Read the model definition and answer for the solid it produces. Units are mm, in the model's axes. A direction names the side the tool comes from. Round coordinates to 2 decimals unless told otherwise and drop trailing zeros. Write each loop counter-clockwise with the first axis right and the second up, starting at its lowest first coordinate (ties: lowest second). Pieces come first, ordered by that corner, then holes. Notation, with made-up numbers: (53, 60) - (92, 60) arc R21 cw to (92, 97) - close; hole circle Ø2 at (-21, 61). An arc over 180 degrees is marked (long way). One line per item, written item: value. Start each with the question number.
(1) A cutting plane is placed at A-A, the plane z = 6.75. Determine the outline of the cut face in (x, y).
(2) Find the intervals of material crossed by L1, parallel to Z at x = -2.5, y = 4; L2, parallel to Y at x = 9, z = 12.5; L3, parallel to Y at x = 12, z = 17.5, in increasing order.
(3) For faces 1 (the face through (5.989, -11.544, 22.712)), 2 (the face through (5.989, 11.544, 22.712)), 3 (the face through (-2.25, 0, 7)), determine the directions among +Z, -Z, +X, -X, +Y, -Y from which every point of the face is accessible in a straight line to the end or side of a thin tool.
(4) A cutting plane is placed at B-B, the plane x = 13. Determine the outline of the cut face in (y, z).
(5) A cutting plane is placed at C-C, the plane z = 11. Determine the outline of the cut face in (x, y).
(6) Flat-ended cylindrical pins translate along their axes: pin 1 Ø1.6 at (y, z) = (-6.5, 23) entering from +X; pin 2 Ø3 at (y, z) = (-4, 7.5) entering from -X; pin 3 Ø6 at (y, z) = (4, 6) entering from +X. Find the tip coordinate at first contact, or state that the pin passes through.
(7) The mould has two halves that part along Z. Classify faces 4 (the face through (12.671, -11.854, 14.79)), 5 (the face through (-5.989, 11.544, 22.712)), 6 (the face through (0, 0, 0)): +Z half, -Z half, draft (parallel to the pull), parting line (faces both ways), or undercut.
(8) A cutting plane is placed at D-D, the plane y = 9.5. Determine the outline of the cut face in (x, z).
from build123d import *

# Parameters (mm, degrees)
F1_DEPTH     = 30
F2_W         = 2.5
F2_H         = 5.5
F3_DEPTH     = 27
F4_T1_DEPTH  = 68.7298334621
F5_T1_DEPTH  = 5.5
F5_T3_DEPTH  = 5.5
F5_T8_DEPTH  = 30.5
F5_T13_DEPTH = 30.5
F5_T18_DEPTH = 30.5
F5_T23_DEPTH = 30.5
F5_T28_DEPTH = 30.5
F5_T33_DEPTH = 30.5
F5_T38_DEPTH = 30.5
F5_T43_DEPTH = 30.5


# Not quite as in the source:
# - a fillet or chamfer that OpenCascade refuses, or shapes differently, is made with other operations: its cross-section is extruded or revolved along the edge and cut away or added


with BuildPart() as f1:
    # F0 (on Top) → F1 (new body)
    with BuildSketch(Plane.XY):
        with BuildLine():
            Line((15.75, 13.25), (-15.75, 13.25))
            Line((-15.75, 13.25), (-15.75, 8.25))
            ThreePointArc((-15.75, 8.25), (-9.9163690552, 5.8336309448), (-7.5, 0))
            ThreePointArc((-7.5, 0), (-9.9163690552, -5.8336309448), (-15.75, -8.25))
            Line((-15.75, -8.25), (-15.75, -13.25))
            Line((-15.75, -13.25), (15.75, -13.25))
            Line((15.75, -13.25), (15.75, -8.25))
            ThreePointArc((15.75, -8.25), (7.5, 0), (15.75, 8.25))
            Line((15.75, 8.25), (15.75, 13.25))
        make_face()
    extrude(amount=F1_DEPTH)

    # F2 (on face) → F3 (cut)
    with BuildSketch(Plane.XZ.offset(13.25)):
        with Locations((-3.5, 22.75)):
            Rectangle(F2_W, F2_H)
        with Locations((-3.5, 7.25)):
            Rectangle(F2_W, F2_H)
        with Locations((3.5, 22.75)):
            Rectangle(F2_W, F2_H)
        with Locations((3.5, 7.25)):
            Rectangle(F2_W, F2_H)
    extrude(amount=-F3_DEPTH, mode=Mode.SUBTRACT)

    # F4: fillet of radius 8.5 on 4 edges, made by hand

    # F4_s2 → F4_t1 (cut)
    with BuildSketch(Plane.XY.offset(-19.364916731)):
        with BuildLine():
            ThreePointArc((-8.0040333076, 13.25), (-12.6138055362, 11.8914284285), (-15.75, 8.25))
            Line((-15.75, 8.25), (-15.75, 13.25))
            Line((-15.75, 13.25), (-8.0040333076, 13.25))
        make_face()
        with BuildLine():
            ThreePointArc((-8.0040333076, -13.25), (-12.6138055362, -11.8914284285), (-15.75, -8.25))
            Line((-15.75, -8.25), (-15.75, -13.25))
            Line((-15.75, -13.25), (-8.0040333076, -13.25))
        make_face()
        with BuildLine():
            ThreePointArc((15.75, -8.25), (12.6138055362, -11.8914284285), (8.0040333076, -13.25))
            Line((8.0040333076, -13.25), (15.75, -13.25))
            Line((15.75, -13.25), (15.75, -8.25))
        make_face()
        with BuildLine():
            ThreePointArc((15.75, 8.25), (12.6138055362, 11.8914284285), (8.0040333076, 13.25))
            Line((8.0040333076, 13.25), (15.75, 13.25))
            Line((15.75, 13.25), (15.75, 8.25))
        make_face()
    extrude(amount=F4_T1_DEPTH, mode=Mode.SUBTRACT)

    # F5: fillet of radius 5 on 8 edges, made by hand

    # F5_s2 → F5_t1 (cut)
    with BuildSketch(Plane.XY.offset(20)):
        with BuildLine():
            ThreePointArc((-9.75, -13.25), (-6.2144660941, -11.7855339059), (-4.75, -8.25))
            Line((-4.75, -8.25), (-4.75, -13.25))
            Line((-4.75, -13.25), (-9.75, -13.25))
        make_face()
        with BuildLine():
            ThreePointArc((9.75, -13.25), (6.2144660941, -11.7855339059), (4.75, -8.25))
            Line((4.75, -8.25), (4.75, -13.25))
            Line((4.75, -13.25), (9.75, -13.25))
        make_face()
        with BuildLine():
            ThreePointArc((9.75, 13.25), (6.2144660941, 11.7855339059), (4.75, 8.25))
            Line((4.75, 8.25), (4.75, 13.25))
            Line((4.75, 13.25), (9.75, 13.25))
        make_face()
        with BuildLine():
            ThreePointArc((-9.75, 13.25), (-6.2144660941, 11.7855339059), (-4.75, 8.25))
            Line((-4.75, 8.25), (-4.75, 13.25))
            Line((-4.75, 13.25), (-9.75, 13.25))
        make_face()
    extrude(amount=F5_T1_DEPTH, mode=Mode.SUBTRACT)

    # F5_s4 → F5_t3 (cut)
    with BuildSketch(Plane.XY.offset(4.5)):
        with BuildLine():
            ThreePointArc((-9.75, -13.25), (-6.2144660941, -11.7855339059), (-4.75, -8.25))
            Line((-4.75, -8.25), (-4.75, -13.25))
            Line((-4.75, -13.25), (-9.75, -13.25))
        make_face()
        with BuildLine():
            ThreePointArc((9.75, -13.25), (6.2144660941, -11.7855339059), (4.75, -8.25))
            Line((4.75, -8.25), (4.75, -13.25))
            Line((4.75, -13.25), (9.75, -13.25))
        make_face()
        with BuildLine():
            ThreePointArc((9.75, 13.25), (6.2144660941, 11.7855339059), (4.75, 8.25))
            Line((4.75, 8.25), (4.75, 13.25))
            Line((4.75, 13.25), (9.75, 13.25))
        make_face()
        with BuildLine():
            ThreePointArc((-9.75, 13.25), (-6.2144660941, 11.7855339059), (-4.75, 8.25))
            Line((-4.75, 8.25), (-4.75, 13.25))
            Line((-4.75, 13.25), (-9.75, 13.25))
        make_face()
    extrude(amount=F5_T3_DEPTH, mode=Mode.SUBTRACT)


with BuildPart() as f5_tool6:
    # F5_s7 → F5_t8 (new body)
    with BuildSketch(Plane.XY.offset(38)):
        with BuildLine():
            ThreePointArc((-9.75, -13.25), (-6.2144660941, -11.7855339059), (-4.75, -8.25))
            Line((-4.75, -8.25), (-4.75, -13.25))
            Line((-4.75, -13.25), (-9.75, -13.25))
        make_face()
    extrude(amount=-F5_T8_DEPTH)

    split(bisect_by=Plane.XY.offset(10), keep=Keep.BOTTOM)


with BuildPart() as f1_1:
    add(f1.part)

    # F5_t5: cut F5_tool6
    add(f5_tool6.part, mode=Mode.SUBTRACT)


with BuildPart() as f5_tool11:
    # F5_s12 → F5_t13 (new body)
    with BuildSketch(Plane.XY.offset(22.5)):
        with BuildLine():
            ThreePointArc((-9.75, -13.25), (-6.2144660941, -11.7855339059), (-4.75, -8.25))
            Line((-4.75, -8.25), (-4.75, -13.25))
            Line((-4.75, -13.25), (-9.75, -13.25))
        make_face()
    extrude(amount=-F5_T13_DEPTH)

    split(bisect_by=Plane.XY.offset(20), keep=Keep.TOP)


with BuildPart() as f1_2:
    add(f1_1.part)

    # F5_t10: cut F5_tool11
    add(f5_tool11.part, mode=Mode.SUBTRACT)


with BuildPart() as f5_tool16:
    # F5_s17 → F5_t18 (new body)
    with BuildSketch(Plane.XY.offset(7.5)):
        with BuildLine():
            ThreePointArc((9.75, -13.25), (6.2144660941, -11.7855339059), (4.75, -8.25))
            Line((4.75, -8.25), (4.75, -13.25))
            Line((4.75, -13.25), (9.75, -13.25))
        make_face()
    extrude(amount=F5_T18_DEPTH)

    split(bisect_by=Plane.XY.offset(10), keep=Keep.BOTTOM)


with BuildPart() as f1_3:
    add(f1_2.part)

    # F5_t15: cut F5_tool16
    add(f5_tool16.part, mode=Mode.SUBTRACT)


with BuildPart() as f5_tool21:
    # F5_s22 → F5_t23 (new body)
    with BuildSketch(Plane.XY.offset(-8)):
        with BuildLine():
            ThreePointArc((9.75, -13.25), (6.2144660941, -11.7855339059), (4.75, -8.25))
            Line((4.75, -8.25), (4.75, -13.25))
            Line((4.75, -13.25), (9.75, -13.25))
        make_face()
    extrude(amount=F5_T23_DEPTH)

    split(bisect_by=Plane.XY.offset(20), keep=Keep.TOP)


with BuildPart() as f1_4:
    add(f1_3.part)

    # F5_t20: cut F5_tool21
    add(f5_tool21.part, mode=Mode.SUBTRACT)


with BuildPart() as f5_tool26:
    # F5_s27 → F5_t28 (new body)
    with BuildSketch(Plane.XY.offset(7.5)):
        with BuildLine():
            ThreePointArc((9.75, 13.25), (6.2144660941, 11.7855339059), (4.75, 8.25))
            Line((4.75, 8.25), (4.75, 13.25))
            Line((4.75, 13.25), (9.75, 13.25))
        make_face()
    extrude(amount=F5_T28_DEPTH)

    split(bisect_by=Plane.XY.offset(10), keep=Keep.BOTTOM)


with BuildPart() as f1_5:
    add(f1_4.part)

    # F5_t25: cut F5_tool26
    add(f5_tool26.part, mode=Mode.SUBTRACT)


with BuildPart() as f5_tool31:
    # F5_s32 → F5_t33 (new body)
    with BuildSketch(Plane.XY.offset(-8)):
        with BuildLine():
            ThreePointArc((9.75, 13.25), (6.2144660941, 11.7855339059), (4.75, 8.25))
            Line((4.75, 8.25), (4.75, 13.25))
            Line((4.75, 13.25), (9.75, 13.25))
        make_face()
    extrude(amount=F5_T33_DEPTH)

    split(bisect_by=Plane.XY.offset(20), keep=Keep.TOP)


with BuildPart() as f1_6:
    add(f1_5.part)

    # F5_t30: cut F5_tool31
    add(f5_tool31.part, mode=Mode.SUBTRACT)


with BuildPart() as f5_tool36:
    # F5_s37 → F5_t38 (new body)
    with BuildSketch(Plane.XY.offset(38)):
        with BuildLine():
            ThreePointArc((-9.75, 13.25), (-6.2144660941, 11.7855339059), (-4.75, 8.25))
            Line((-4.75, 8.25), (-4.75, 13.25))
            Line((-4.75, 13.25), (-9.75, 13.25))
        make_face()
    extrude(amount=-F5_T38_DEPTH)

    split(bisect_by=Plane.XY.offset(10), keep=Keep.BOTTOM)


with BuildPart() as f1_7:
    add(f1_6.part)

    # F5_t35: cut F5_tool36
    add(f5_tool36.part, mode=Mode.SUBTRACT)


with BuildPart() as f5_tool41:
    # F5_s42 → F5_t43 (new body)
    with BuildSketch(Plane.XY.offset(22.5)):
        with BuildLine():
            ThreePointArc((-9.75, 13.25), (-6.2144660941, 11.7855339059), (-4.75, 8.25))
            Line((-4.75, 8.25), (-4.75, 13.25))
            Line((-4.75, 13.25), (-9.75, 13.25))
        make_face()
    extrude(amount=-F5_T43_DEPTH)

    split(bisect_by=Plane.XY.offset(20), keep=Keep.TOP)


with BuildPart() as f1_8:
    add(f1_7.part)

    # F5_t40: cut F5_tool41
    add(f5_tool41.part, mode=Mode.SUBTRACT)


solid = f1_8.part
Here are the results:
1. outline: (-15.75, -8.25) arc R8.5 ccw to (-8.99, -13.19) arc R5 ccw to (-4.75, -8.25) - (-4.75, 8.25) arc R5 ccw to (-8.99, 13.19) arc R8.5 ccw to (-15.75, 8.25) arc R8.25 cw to start; (-2.25, -13.25) - (2.25, -13.25) - (2.25, 13.25) - (-2.25, 13.25) - close; (4.75, -8.25) arc R5 ccw to (8.99, -13.19) arc R8.5 ccw to (15.75, -8.25) arc R8.25 cw to (15.75, 8.25) arc R8.5 ccw to (8.99, 13.19) arc R5 ccw to (4.75, 8.25) - close
2. L1: 0 to 4.5, 10 to 20, 25.5 to 30
2. L2: -13.19 to -4.74, 4.74 to 13.19
2. L3: -12.25 to -7.35, 7.35 to 12.25
3. face 1: -Y
3. face 2: +Y
3. face 3: +Y, -Y
4. outline: (-11.63, 0) - (-7.78, 0) - (-7.78, 30) - (-11.63, 30) - close; (7.78, 0) - (11.63, 0) - (11.63, 30) - (7.78, 30) - close
5. outline: (-15.75, -8.25) arc R8.5 ccw to (-8, -13.25) - (8, -13.25) arc R8.5 ccw to (15.75, -8.25) arc R8.25 cw to (15.75, 8.25) arc R8.5 ccw to (8, 13.25) - (-8, 13.25) arc R8.5 ccw to (-15.75, 8.25) arc R8.25 cw to start
6. pin 1: x = 11.91
6. pin 2: x = -9.6
6. pin 3: x = 11.38
7. face 4: draft
7. face 5: undercut
7. face 6: -Z half
8. outline: (-15.05, 0) - (15.05, 0) - (15.05, 30) - (-15.05, 30) - close; hole (-4.91, 4.5) - (-2.25, 4.5) - (-2.25, 10) - (-4.91, 10) - close; hole (-4.91, 20) - (-2.25, 20) - (-2.25, 25.5) - (-4.91, 25.5) - close; hole (2.25, 4.5) - (4.91, 4.5) - (4.91, 10) - (2.25, 10) - close; hole (2.25, 20) - (4.91, 20) - (4.91, 25.5) - (2.25, 25.5) - close
